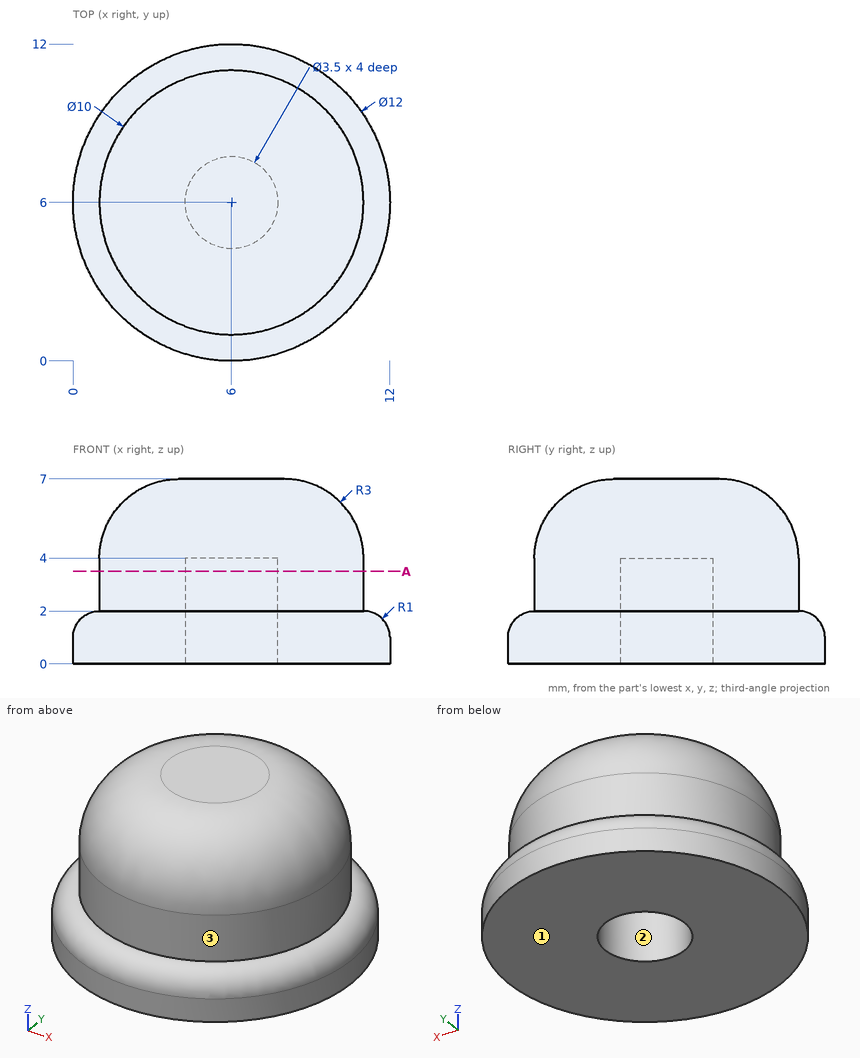
Part print with two shaded views. Sizes in mm from the minimum x, y, z corner. Give positions to 0.01 mm unless a question says otherwise; leave off trailing zeros. Order: outer loops, then holes, each group sorted by start corner. A loop starts at its lowest first (then second) coordinate and runs counter-clockwise, first axis right, second up. Notation, with made-up numbers: M 69,-34.75 L 121,-34.75 A13 ccw 121,-23.75 Z; hole C -21.5,-2.5 d9. An arc over 180 degrees is marked long. Put each result on its own line as item: value.
Item 1: Drop flat-ended pins along their axis: pin 1 Ø1 at (x, z) = (8, 2) entering from +Y; pin 2 Ø1 at (y, z) = (8.5, 5.5) entering from +X; pin 3 Ø1.5 at (x, y) = (6, 5.5) entering from -Z; pin 4 Ø1 at (x, y) = (9, 4.5) entering from -Z. Give the stop position or say it passes through.
Results are:
pin 1: y = 11.56
pin 2: x = 10.26
pin 3: z = 4
pin 4: z = 0
Item 2: Cut at A-A on z = 3.5. Write the cut outline in (x, y).
Results are:
outline: C 6,6 d10; hole C 6,6 d3.5
Item 3: Pull direction X, two halves, no side cores. Call the marked faces 1, 2 and 3: +X half, -X half, draft (parallel to the pull), parting line (faces both ways), or undercut.
Results are:
face 1: draft
face 2: undercut
face 3: parting line
Item 4: Wall check: probe 1 along Y at (x, z) = (6, 0.9); probe 2 along Z at (x, y) = (6.25, 7.25); probe 3 along X at (y, z) = (6, 1.1) (3 decimals). Give the ranges that are in metal, low to high.
Results are:
probe 1: 0 to 4.25, 7.75 to 12
probe 2: 4 to 7
probe 3: 0.005 to 4.25, 7.75 to 11.995
